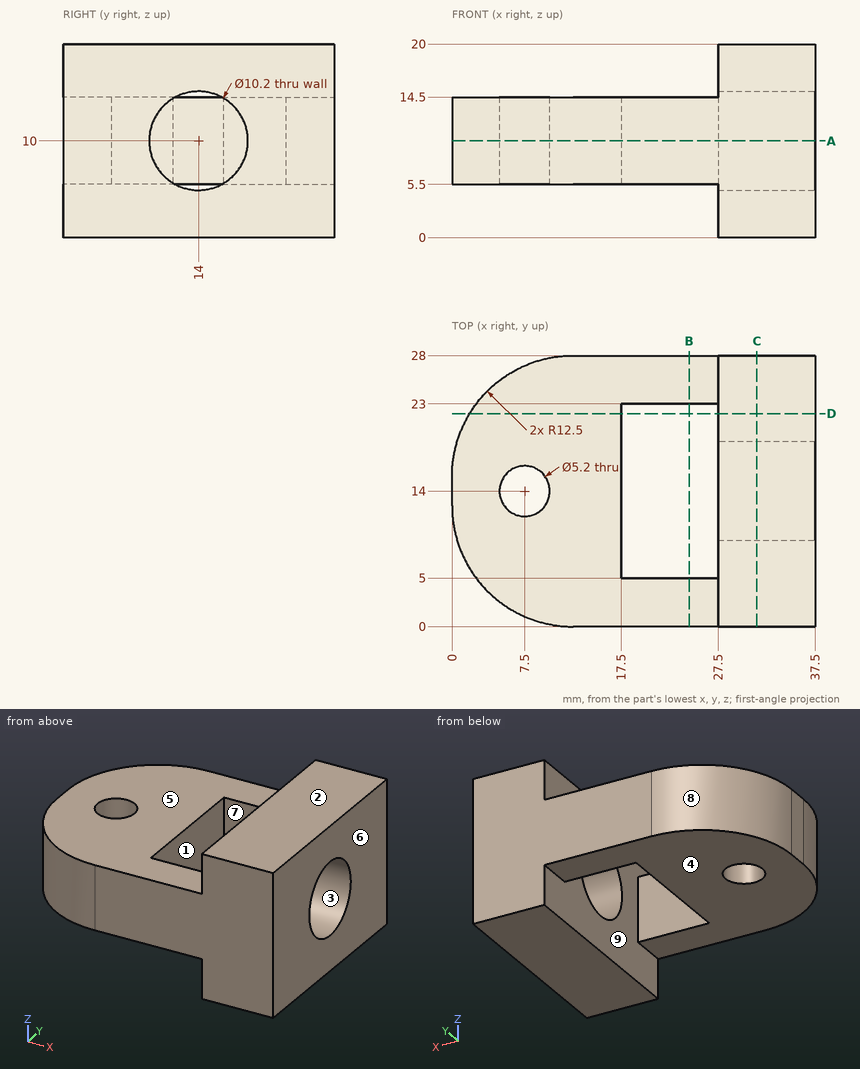
Study the drawing (mm; zero at the part's minimum x, y, z) and answer. A direction names the side the tool comes from. Round coordinates to 2 decimals unless told otherwise and drop trailing zeros. Write each loop counter-clockwise with the first axis right and the second up, starting at its lowest first coordinate (ties: lowest second). Pieces come first, ordered by that corner, then holes. Notation, with made-up numbers: (40, 27) - (80, 27) arc R14 ccw to (80, 54) - close; hole circle Ø6 at (32.25, 1). An arc over 180 degrees is marked (long way). Use a Markdown table: item, result. Add a question column.
1. For a pull along Z with two mould halves and no side action, classify the marked faces 1, 2, 3 and 4 as +Z half, -Z half, draft (parallel to the pull), parting line (faces both ways), or undercut.
2. Flat-ended cylindrical pins translate along their axes: P1, Ø1.5, axis at x = 7, y = 12, coming from the -Z side; P2, Ø3, axis at x = 4.5, y = 10.5, coming from the +Z side; P3, Ø1.5, axis at y = 24, z = 4.5, coming from the -X side. Find the tip coordinate at first contact, or state that the pin passes through.
3. Consider line 1 (Z direction, x = 31.25, y = 14); line 2 (Y direction, x = 34, z = 10.25); line 3 (Z direction, x = 16, y = 3). Determine where each line is inside the solid, lowest interval first.
4. The part is cut by section C-C (x = 31.5). Write down the section's boundary in (y, z), and give its area (3 significant figures).
5. The part is cut by section B-B (x = 24.5). Write down the section's boundary in (y, z).
6. The part is cut by section D-D (y = 22). Write down the section's boundary in (x, z), and give its area (3 significant figures).
7. The part is cut by section A-A (z = 10). Write down the section's boundary in (x, y), and give its area (3 significant figures).
8. A tool of negligible diameter and unlimited length cuts with its end or side. For the marked faces 5, 6, 7, 8 and 9, from which of +Z, -Z, +X, -X, +Y, -Y can it reach the whole face along a straight path? Write none if from no direction.
Reported:
| question | item | result |
|---|---|---|
| 1 | face 1 | draft |
| 1 | face 2 | +Z half |
| 1 | face 3 | undercut |
| 1 | face 4 | -Z half |
| 2 | P1 | z = 5.5 |
| 2 | P2 | z = 14.5 |
| 2 | P3 | x = 27.5 |
| 3 | line 1 | 0 to 4.9, 15.1 to 20 |
| 3 | line 2 | 0 to 8.91, 19.09 to 28 |
| 3 | line 3 | 5.5 to 14.5 |
| 4 | outline | (0, 0) - (28, 0) - (28, 20) - (0, 20) - close; hole circle Ø10.2 at (14, 10) |
| 4 | area | 478 mm^2 |
| 5 | outline | (0, 5.5) - (5, 5.5) - (5, 14.5) - (0, 14.5) - close; (23, 5.5) - (28, 5.5) - (28, 14.5) - (23, 14.5) - close |
| 6 | outline | (1.82, 5.5) - (17.5, 5.5) - (17.5, 14.5) - (1.82, 14.5) - close; (27.5, 0) - (37.5, 0) - (37.5, 20) - (27.5, 20) - close |
| 6 | area | 341 mm^2 |
| 7 | outline | (0, 12.5) arc R12.5 ccw to (12.5, 0) - (37.5, 0) - (37.5, 8.9) - (27.5, 8.9) - (27.5, 5) - (17.5, 5) - (17.5, 23) - (27.5, 23) - (27.5, 19.1) - (37.5, 19.1) - (37.5, 28) - (12.5, 28) arc R12.5 ccw to (0, 15.5) - close; hole circle Ø5.2 at (7.5, 14) |
| 7 | area | 680 mm^2 |
| 8 | face 5 | +Z, -X, +Y, -Y |
| 8 | face 6 | +Z, -Z, +X, +Y, -Y |
| 8 | face 7 | +Z, -Z |
| 8 | face 8 | +Z, -Z, -X, +Y |
| 8 | face 9 | none |
